```python
from build123d import *

# Parameters (mm, degrees)
F0_W     = 85.725
F0_H     = 76.2
F1_DEPTH = 19.05
F2_R     = 25.4
F3_DEPTH = 25.4
F5_DEPTH = 25.4


with BuildPart() as f1:
    # F0 (on Front) → F1 (new body)
    with BuildSketch(Plane.XZ):
        with Locations((42.8625, 38.1)):
            Rectangle(F0_W, F0_H)
    extrude(amount=F1_DEPTH)

    # F2 (on face) → F3 (cut)
    with BuildSketch(Plane.XZ.offset(19.05)):
        with Locations((38.1, 38.1)):
            Circle(F2_R)
    extrude(amount=-F3_DEPTH, mode=Mode.SUBTRACT)

    # F4 (on face) → F5 (cut)
    with BuildSketch(Plane.XZ.offset(19.05)):
        Polygon((85.725, 12.7), (85.725, 22.225), (57.927869, 22.225), (38.1, 12.7), align=None)
    extrude(amount=-F5_DEPTH, mode=Mode.SUBTRACT)


solid = f1.part
```
Input: part model. Units: mm. Frame: model coordinates. A direction names the side the tool comes from. Coordinates: 2 decimals unless noted, no trailing zeros. Order: outer loops, then holes, each group sorted by start corner. A loop starts at its lowest first (then second) coordinate and runs counter-clockwise, first axis right, second up. Notation, with made-up numbers: (-37.5, 61.5) - (-1.5, 61.5) arc R22 cw to (-1.5, 89.5) - close; hole circle Ø2 at (28, 29). An arc over 180 degrees is marked (long way). Return JSON: item names as keys, results as strings.
Q1. Draft query along Z for faces 1 (the flat face through (85.725, -9, 49)), 2 (the cylindrical face through (27.973, -9.658, 61.394)), 3 (the flat face through (42, -9, 0)). Return one class per face: +Z half, -Z half, draft (parallel to the pull), parting line (faces both ways), or undercut.
The answers:
{"face 1": "draft", "face 2": "undercut", "face 3": "-Z half"}
Q2. Cut plane A-A (z = 56.5). Return loops of the section in (x, y) (3 decimals), then the cut area to 3 significant figures.
The answers:
{"outline": "(0, -19.05) - (20.59, -19.05) - (20.59, 0) - (0, 0) - close; (55.61, -19.05) - (85.725, -19.05) - (85.725, 0) - (55.61, 0) - close", "area": "966 mm2"}
Q3. Ray query, probe 1 along Z at (x, y) = (38.1, -5); probe 2 along Z at (x, y) = (74, -7.5) (3 decimals); probe 3 along X at (y, z) = (-4.75, 38.1) (3 decimals). Return the intervals inside material, ascending.
The answers:
{"probe 1": "z = 0 to 12.7, 63.5 to 76.2", "probe 2": "z = 0 to 12.7, 22.225 to 76.2", "probe 3": "x = 0 to 12.7, 63.5 to 85.725"}
Q4. Cut plane D-D (z = 20.5). Return loops of the section in (x, y), then the cut area to 3 significant figures.
The answers:
{"outline": "(0, -19.05) - (19.79, -19.05) - (19.79, 0) - (0, 0) - close", "area": "377 mm2"}
Q5. First-contact query: pin 1 (10 mm diameter, centred on y = -9.5, z = 15, fed in from +X) (3 decimals). Flat tip, straight axial feed; report the tip coordinate or a pass-through.
The answers:
{"pin 1": "stops at x = 85.725"}
Q6. Cut plane B-B (x = 73.5). Return loops of the section in (y, z) (3 decimals), then the cut area to 3 significant figures.
The answers:
{"outline": "(-19.05, 0) - (0, 0) - (0, 12.7) - (-19.05, 12.7) - close; (-19.05, 22.225) - (0, 22.225) - (0, 76.2) - (-19.05, 76.2) - close", "area": "1,270 mm2"}
Q7. Cut plane C-C (y = -6.25). Return loops of the section in (x, z) (3 decimals).
The answers:
{"outline": "(0, 0) - (85.725, 0) - (85.725, 12.7) - (38.1, 12.7) arc R25.4 cw (long way) to (57.928, 22.225) - (85.725, 22.225) - (85.725, 76.2) - (0, 76.2) - close"}
Q8. Access query for faces 4 (the flat face through (0, -9, 38)), 5 (the flat face through (62, -10, 12.7)). Directions: +Z, -Z, +X, -X, +Y, -Y. A direction counts if a zero-diameter tool reaches every point of the face in a straight line with its end or side. Return the directions, or none.
The answers:
{"face 4": "+Z, -Z, -X, +Y, -Y", "face 5": "+X, +Y, -Y"}
